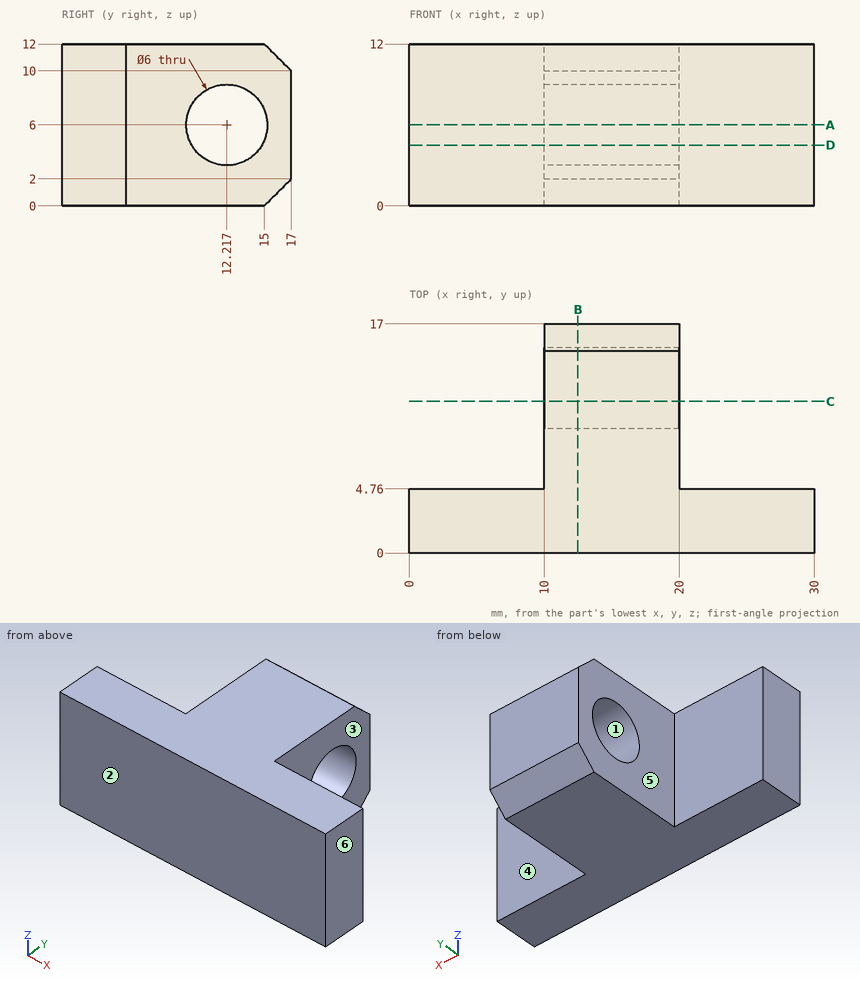
Here's the drawing with two shaded views (mm, measured from the low corner). I have some questions. A direction names the side the tool comes from. Round coordinates to 2 decimals unless told otherwise and drop trailing zeros. Loops run counter-clockwise (first coordinate to the right, second up) from the corner with the lowest first, then second, coordinate; pieces in that order, holes last. Notation, with made-up numbers: M -18,47 L 39,47 A22 cw 39,60 Z; hole C 82.5,-19.75 d1. An arc over 180 degrees is marked long. Answer as CSV lines item,"result".
1) We'd pull the mould along Y, two halves only. Please class the marked faces 1, 2, 3 and 4: released by +Y, released by -Y, zero draft, split by the parting line, or undercut.
From the geometry:
face 1,"undercut"
face 2,"released by -Y"
face 3,"zero draft"
face 4,"released by +Y"
2) Imagine slicing it at C-C on y = 11.25. List the corners of the cut face in (x, z) for me.
From the geometry:
outline,"M 10,0 L 20,0 L 20,3.16 L 10,3.16 Z; M 10,8.84 L 20,8.84 L 20,12 L 10,12 Z"
3) Imagine slicing it at B-B on x = 12.5. List the corners of the cut face in (y, z) for me, and give its area (3 significant figures).
From the geometry:
outline,"M 0,0 L 15,0 L 17,2 L 17,10 L 15,12 L 0,12 Z; hole C 12.22,6 d6"
area,"172 mm^2"
4) Imagine slicing it at D-D on z = 4.5. List the corners of the cut face in (x, y) for me (3 decimals), and give its area (3 significant figures).
From the geometry:
outline,"M 0,0 L 30,0 L 30,4.76 L 20,4.76 L 20,9.619 L 10,9.619 L 10,4.76 L 0,4.76 Z; M 10,14.815 L 20,14.815 L 20,17 L 10,17 Z"
area,"213 mm^2"
5) For pin 1 Ø10 at (x, y) = (22, 9) entering from -Z; pin 2 Ø2 at (x, z) = (24.5, 8.5) entering from +Y; pin 3 Ø5 at (y, z) = (12.22, 6) entering from -X; pin 4 Ø2 at (y, z) = (13.5, 3.5) entering from +X, each with a flat end and sliding along its axis, tell me the tip position at first contact or that it passes through.
From the geometry:
pin 1,"z = 0"
pin 2,"y = 4.76"
pin 3,"through"
pin 4,"x = 20"
6) Imagine slicing it at A-A on z = 6. List the corners of the cut face in (x, y) for me, and give its area (3 significant figures).
From the geometry:
outline,"M 0,0 L 30,0 L 30,4.76 L 20,4.76 L 20,9.22 L 10,9.22 L 10,4.76 L 0,4.76 Z; M 10,15.22 L 20,15.22 L 20,17 L 10,17 Z"
area,"205 mm^2"
7) If I drill on probe 1 along Y at (x, z) = (12.5, 6); probe 2 along X at (y, z) = (9.25, 4.5); probe 3 along Z at (x, y) = (16.5, 13.5), over which ranges is the centre line in solid material (lowest first)?
From the geometry:
probe 1,"0 to 9.22, 15.22 to 17"
probe 2,"10 to 20"
probe 3,"0 to 3.29, 8.71 to 12"
8) Which directions (+Z, -Z, +X, -X, +Y, -Y) give clear straight access to the entire face, cutting with the end or side of a thin tool? Please do the marked faces 5 and 6.
From the geometry:
face 5,"+Z, -Z, -X, +Y"
face 6,"+Z, -Z, +X, +Y, -Y"
